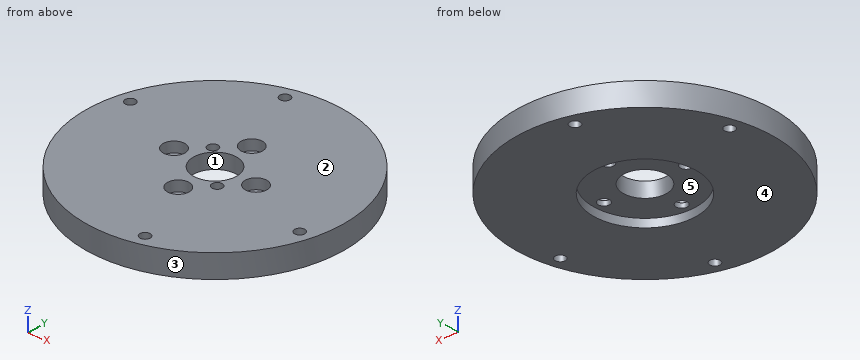
```python
from build123d import *

# Parameters (mm, degrees)
SKETCH_1_R          = 25
SKETCH_1_R_2        = 2.3
SKETCH_1_R_3        = 1.1
SKETCH_1_R_4        = 1
EXTRUDE_1_DEPTH     = 4.5
SKETCH_2_R          = 2.1
CUT_EXTRUDE_1_DEPTH = 2
SKETCH_10_R         = 10
CUT_EXTRUDE_7_DEPTH = 1.6
SKETCH_9_R          = 4.2
CUT_EXTRUDE_5_DEPTH = 36.474075041
SKETCH_6_R          = 1
CUT_EXTRUDE_6_DEPTH = 2


with BuildPart() as part:
    # 스케치1 → 보스-돌출1 (new body)
    with BuildSketch(Plane.XY):
        Circle(SKETCH_1_R)
        Circle(SKETCH_1_R_2, mode=Mode.SUBTRACT)
        with Locations((0, 8)):
            Circle(SKETCH_1_R_3, mode=Mode.SUBTRACT)
        with Locations((8, 0)):
            Circle(SKETCH_1_R_3, mode=Mode.SUBTRACT)
        with Locations((0, -8)):
            Circle(SKETCH_1_R_3, mode=Mode.SUBTRACT)
        with Locations((-8, 0)):
            Circle(SKETCH_1_R_3, mode=Mode.SUBTRACT)
        with Locations((-5.823428515, 21.733331092)):
            Circle(SKETCH_1_R_4, mode=Mode.SUBTRACT)
        with Locations(Location((21.733331092, -5.823428515, 0), (0, 0, 180))):
            Circle(SKETCH_1_R_4, mode=Mode.SUBTRACT)
        with Locations((5.823428515, -21.733331092)):
            Circle(SKETCH_1_R_4, mode=Mode.SUBTRACT)
        with Locations(Location((-21.733331092, 5.823428515, 0), (0, 0, 180))):
            Circle(SKETCH_1_R_4, mode=Mode.SUBTRACT)
    extrude(amount=EXTRUDE_1_DEPTH)

    # 스케치2 → 컷-돌출1 (cut)
    with BuildSketch(Plane.XY.offset(4.5)):
        with Locations((0, 8)):
            Circle(SKETCH_2_R)
        with Locations((8, 0)):
            Circle(SKETCH_2_R)
        with Locations((0, -8)):
            Circle(SKETCH_2_R)
        with Locations((-8, 0)):
            Circle(SKETCH_2_R)
    extrude(amount=-CUT_EXTRUDE_1_DEPTH, mode=Mode.SUBTRACT)

    # 스케치10 → 컷-돌출7 (cut)
    with BuildSketch(Plane(origin=(0, 0, 0), x_dir=(-1, 0, 0), z_dir=(0, 0, -1))):
        Circle(SKETCH_10_R)
    extrude(amount=-CUT_EXTRUDE_7_DEPTH, mode=Mode.SUBTRACT)

    # 스케치9 → 컷-돌출5 (cut, through all)
    with BuildSketch(Plane(origin=(0, 0, 1.6), x_dir=(-1, 0, 0), z_dir=(0, 0, -1))):
        Circle(SKETCH_9_R)
    extrude(amount=-CUT_EXTRUDE_5_DEPTH, mode=Mode.SUBTRACT)

    # 스케치6 → 컷-돌출6 (cut)
    with BuildSketch(Plane.XY.offset(4.5)):
        with Locations((-3.959797975, 3.959797975)):
            Circle(SKETCH_6_R)
        with Locations((3.959797975, -3.959797975)):
            Circle(SKETCH_6_R)
    extrude(amount=-CUT_EXTRUDE_6_DEPTH, mode=Mode.SUBTRACT)


solid = part.part
```
For this review, take the finished solid that the model builds, in its own axes (mm). Face numbers are marked on the shaded views. A direction names the side the tool comes from. Coordinates: 2 decimals unless noted, no trailing zeros. Loops run counter-clockwise (first coordinate to the right, second up) from the corner with the lowest first, then second, coordinate; pieces in that order, holes last.
1. Add section A-A, the plane x = 0. Give the boundary of the cut face in (y, z), then the cut area to 3 significant figures.
2. For line 1 (X direction, y = 3.5, z = 3.55); line 2 (Y direction, x = 0, z = 0.35); line 3 (X direction, y = 5.5, z = 0.85), list the stretches that pass through material, from the lowest coordinate up.
3. Insertion check: P1, Ø1.6, axis at x = 3.96, y = -3.96, coming from the -Z side; P2, Ø2, axis at y = -7, z = 2.5, coming from the -X side; P3, Ø1, axis at y = 12.5, z = 2.5, coming from the -X side. Each pin has a flat end and moves straight along its axis. Give the tip position at first contact, or say it passes through.
4. For the marked faces 4 and 5, list the 3-axis set-ups (+Z, -Z, +X, -X, +Y, -Y) from which the entire face can be reached by the end or side of a thin tool; tool diameter is ignored.
5. Add section B-B, the plane y = -8. Give the boundary of the cut face in (x, z).
6. Mouldability with a two-part tool opening along Y and no side actions: class the marked faces 1, 2 and 3 as +Y half, -Y half, draft (parallel to the pull), parting line (faces both ways), or undercut.
Result:
1. outline: (-25, 0) - (-10, 0) - (-10, 1.6) - (-9.1, 1.6) - (-9.1, 2.5) - (-10.1, 2.5) - (-10.1, 4.5) - (-25, 4.5) - close; (-6.9, 1.6) - (-4.2, 1.6) - (-4.2, 4.5) - (-5.9, 4.5) - (-5.9, 2.5) - (-6.9, 2.5) - close; (4.2, 1.6) - (6.9, 1.6) - (6.9, 2.5) - (5.9, 2.5) - (5.9, 4.5) - (4.2, 4.5) - close; (9.1, 1.6) - (10, 1.6) - (10, 0) - (25, 0) - (25, 4.5) - (10.1, 4.5) - (10.1, 2.5) - (9.1, 2.5) - close
1. area: 148 mm2
2. line 1: x = -24.75 to -4.85, -3.07 to -2.32, 2.32 to 24.75
2. line 2: y = -25 to -10, 10 to 25
2. line 3: x = -24.39 to -22.68, -20.79 to -8.35, 8.35 to 24.39
3. P1: stops at z = 1.6
3. P2: stops at x = -24.27
3. P3: stops at x = -21.93
4. face 4: -Z, +X, -X, +Y, -Y
4. face 5: -Z
5. outline: (-23.69, 0) - (-6, 0) - (-6, 1.6) - (-1.1, 1.6) - (-1.1, 2.5) - (-2.1, 2.5) - (-2.1, 4.5) - (-23.69, 4.5) - close; (1.1, 1.6) - (6, 1.6) - (6, 0) - (23.69, 0) - (23.69, 4.5) - (2.1, 4.5) - (2.1, 2.5) - (1.1, 2.5) - close
6. face 1: undercut
6. face 2: draft
6. face 3: parting line
